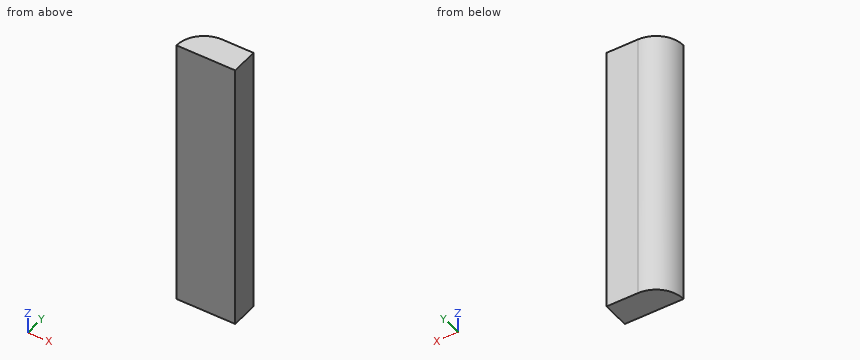
Autodesk Inventor part; units mm, degrees
ref_plane "YZ Plane" through (0, 0, 0) normal (1, 0, 0) x (0, 1, 0)
ref_plane "XZ Plane" through (0, 0, 0) normal (0, 1, 0) x (-1, 0, 0)
ref_plane "XY Plane" through (0, 0, 0) normal (0, 0, 1) x (1, 0, 0)
sketch "Sketch1" plane through (0, 0, 0) normal (0, 1, 0) x (-1, 0, 0)
  line L0 (24.6138, 28.8821) -> (9.6138, 28.8821)
  line L1 (9.6138, 28.8821) -> (9.6138, -41.1179)
  line L2 (9.6138, -41.1179) -> (24.6138, -41.1179)
  line L3 (24.6138, -41.1179) -> (24.6138, 28.8821)
  point P0 (0, 0)
  dimension "d0" = 70
  dimension "d1" = 15
extrude "Extrusion1" add sketch "Sketch1" along normal blind 7
fillet "Fillet1" radius 7 1 edges at (-24.6138, 7, -6.1179)
properties part number "Paper-holder-clip" material "Steel"
Geometry: final body of the model. Coordinates: model frame, mm. Round coordinates to 2 decimals unless told otherwise and drop trailing zeros. Write each loop counter-clockwise with the first axis right and the second up, starting at its lowest first coordinate (ties: lowest second). Pieces come first, ordered by that corner, then holes. Notation, with made-up numbers: (-12, 17.25) -> (-7, 17.25) arc R5 ccw to (-7, 21.25) -> close; hole circle Ø3 at (-35.75, -28.5). An arc over 180 degrees is marked (long way). Use CSV: the item, a comma, the result in double quotes. Start each with the question number.
Q1. First-contact query: pin 1 Ø4 at (x, z) = (-21.5, -24) entering from +Y; pin 2 Ø3 at (x, z) = (-21.5, -23.5) entering from +Y. Flat tips, straight axial feed; report the tip coordinate or a pass-through.
Q2. Line query: L1, parallel to Y at x = -18, z = -35; L2, parallel to X at y = 3.5, z = 12; L3, parallel to X at y = 5.75, z = -25. Output: solid intervals per line, ascending.
Q3. Section C-C (x = -19.5). Return loops of the section in (y, z), plus the area to 3 significant figures.
Q4. Section B-B (y = 5.75). Return loops of the section in (x, z).
Result sheet:
1,pin 1,"y = 6.74"
1,pin 2,"y = 6.58"
2,L1,"0 to 6.99"
2,L2,"-23.68 to -9.61"
2,L3,"-21.61 to -9.61"
3,outline,"(0, -41.12) -> (6.74, -41.12) -> (6.74, 28.88) -> (0, 28.88) -> close"
3,area,"472 mm²"
4,outline,"(-21.61, -41.12) -> (-9.61, -41.12) -> (-9.61, 28.88) -> (-21.61, 28.88) -> close"
